Can you work these out from the drawing? Everything is in mm from the part's minimum corner. A direction names the side the tool comes from. Coordinates: 2 decimals unless noted, no trailing zeros. Loops run counter-clockwise (first coordinate to the right, second up) from the corner with the lowest first, then second, coordinate; pieces in that order, holes last.
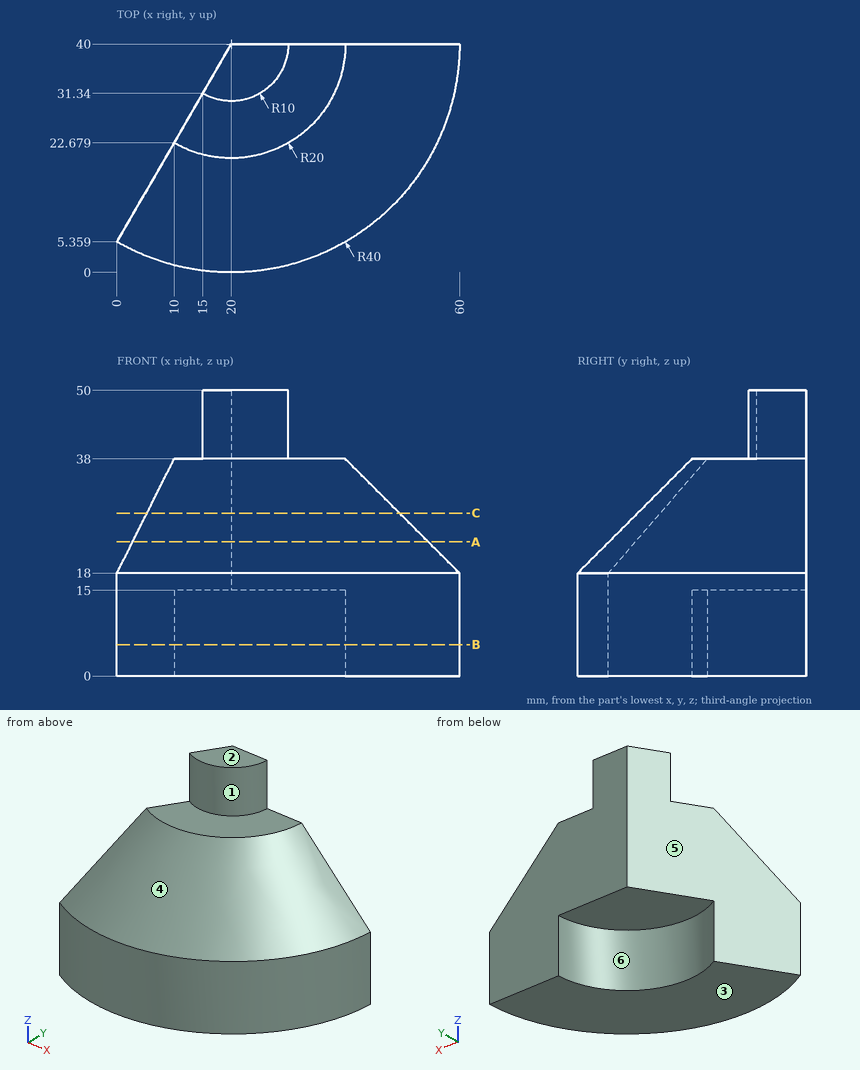
Item 1: I'm going to push flat-ended pins straight in: P1, Ø4, axis at x = 32.5, z = 29, coming from the -Y side; P2, Ø8, axis at y = 22.5, z = 21.5, coming from the -X side; P3, Ø8, axis at y = 27.5, z = 33, coming from the +X side; P4, Ø3, axis at y = 17.5, z = 38, coming from the +X side. Where does each tip first touch, or does it pass through?
Results are:
P1: stops at y = 11.47
P2: stops at x = 7.59
P3: stops at x = 46.52
P4: passes through
Item 2: Suppose I cut it at B-B, the plane z = 5.5. Please give me the cut outline in (x, y), plus the area to 3 significant figures.
Results are:
outline: (0, 5.36) arc R40 ccw to (60, 40) - (40, 40) arc R20 cw to (10, 22.68) - close
area: 1,260 mm2
Item 3: Suppose I cut it at A-A, the plane z = 23.5. Please give me the cut outline in (x, y).
Results are:
outline: (2.75, 10.12) arc R34.5 ccw to (54.5, 40) - (20, 40) - close
Item 4: Suppose I cut it at C-C, the plane z = 28.5. Please give me the cut outline in (x, y), plus the area to 3 significant figures.
Results are:
outline: (5.25, 14.45) arc R29.5 ccw to (49.5, 40) - (20, 40) - close
area: 911 mm2
Item 5: On a 3-axis mill with a long thin cutter (end or side, diameter ignored), from which of +Z, -Z, +X, -X, +Y, -Y can I reach the whole of each face in a straight line? I mean the marked faces 1 and 2. Say none if no direction works.
Results are:
face 1: +Z, -Y
face 2: +Z, +X, -X, +Y, -Y
Item 6: I need wall thicknesses on line 1 along X through (y, z) = (22, 11) (1 decimal); line 2 along Y through (x, z) = (29, 47) (1 decimal); line 3 along X through (y, z) = (32, 11.5). Which ranges of each line are inside material? Lowest first, please.
Results are:
line 1: x = 9.6 to 11.3, 28.7 to 55.7
line 2: y = 35.6 to 40
line 3: x = 38.33 to 59.19
Item 7: We'd pull the mould along X, two halves only. Please class the marked faces 3, 4, 5 and 6: +X half, -X half, draft (parallel to the pull), parting line (faces both ways), or undercut.
Results are:
face 3: draft
face 4: parting line
face 5: -X half
face 6: undercut
